Could you check a few things on this drawing? It's one solid part, dimensions in mm from its lowest x, y, z. Give positions to 0.01 mm unless a question says otherwise; leave off trailing zeros. Order: outer loops, then holes, each group sorted by start corner. A loop starts at its lowest first (then second) coordinate and runs counter-clockwise, first axis right, second up. Notation, with made-up numbers: (-20, 25) - (38, 25) arc R36 cw to (38, 61) - close; hole circle Ø10 at (88, 33). An arc over 180 degrees is marked (long way). Answer as CSV lines item,"result".
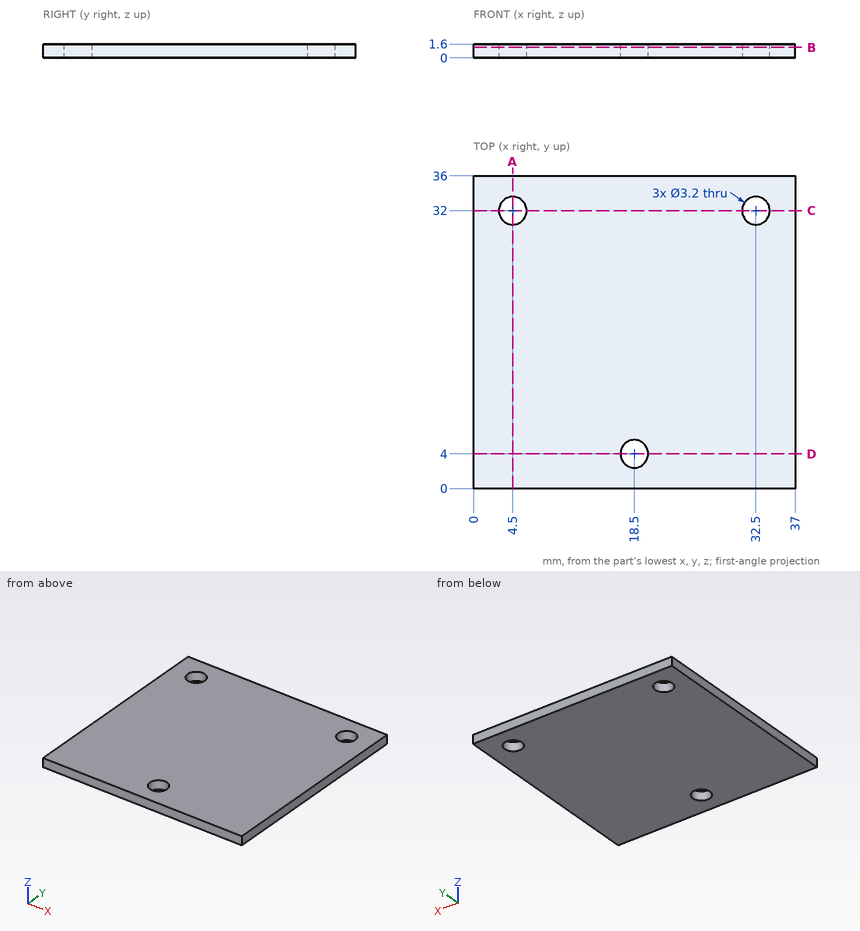
1) I want a section at A-A on x = 4.5. Write out the boundary of the cut face in (y, z).
Answer block:
outline,"(0, 0) - (30.4, 0) - (30.4, 1.6) - (0, 1.6) - close; (33.6, 0) - (36, 0) - (36, 1.6) - (33.6, 1.6) - close"
2) I want a section at C-C on y = 32. Write out the boundary of the cut face in (x, z).
Answer block:
outline,"(0, 0) - (2.9, 0) - (2.9, 1.6) - (0, 1.6) - close; (6.1, 0) - (30.9, 0) - (30.9, 1.6) - (6.1, 1.6) - close; (34.1, 0) - (37, 0) - (37, 1.6) - (34.1, 1.6) - close"
3) I need wall thicknesses on line 1 along Y through (x, z) = (18.5, 1.2); line 2 along X through (y, z) = (32.5, 0.75); line 3 along Y through (x, z) = (4.5, 0.6). Which ranges of each line are inside material? Lowest first, please. Write a range as [from, to].
Answer block:
line 1,"[0, 2.4], [5.6, 36]"
line 2,"[0, 2.98], [6.02, 30.98], [34.02, 37]"
line 3,"[0, 30.4], [33.6, 36]"
4) I want a section at D-D on y = 4. Write out the boundary of the cut face in (x, z), plus the area to 3 significant figures.
Answer block:
outline,"(0, 0) - (16.9, 0) - (16.9, 1.6) - (0, 1.6) - close; (20.1, 0) - (37, 0) - (37, 1.6) - (20.1, 1.6) - close"
area,"54.1 mm2"
5) I want a section at B-B on z = 1.2. Write out the boundary of the cut face in (x, y).
Answer block:
outline,"(0, 0) - (37, 0) - (37, 36) - (0, 36) - close; hole circle Ø3.2 at (4.5, 32); hole circle Ø3.2 at (18.5, 4); hole circle Ø3.2 at (32.5, 32)"
6) I'm going to push a flat-ended pin straight in: P1, Ø4, axis at x = 18.5, y = 4, coming from the +Z side. Where does the tip first touch, or does it pass through?
Answer block:
P1,"z = 1.6"
